Can you work these out from the model? Positions are in its coordinate system, mm. A direction names the side the tool comes from. Round coordinates to 2 decimals unless told otherwise and drop trailing zeros. Order: outer loops, then holes, each group sorted by start corner. A loop starts at its lowest first (then second) coordinate and runs counter-clockwise, first axis right, second up.
from build123d import *

# Parameters (mm, degrees)
SKETCH1_W           = 150
SKETCH1_H           = 20
BOSS_EXTRUDE1_DEPTH = 5
SKETCH3_W           = 150
SKETCH3_H           = 5
BOSS_EXTRUDE2_DEPTH = 15
SKETCH5_R           = 2
CUT_EXTRUDE1_DEPTH  = 152.492574075
SKETCH6_R           = 1.75
CUT_EXTRUDE2_DEPTH  = 153.069063257
SKETCH7_W           = 5
SKETCH7_H           = 20
BOSS_EXTRUDE3_DEPTH = 17
SKETCH8_R           = 1.5
CUT_EXTRUDE3_DEPTH  = 152.492574075
FILLET2_R           = 15


with BuildPart() as part:
    # Sketch1 → Boss-Extrude1 (new body)
    with BuildSketch(Plane(origin=(0, 0, 0), x_dir=(1, 0, 0), z_dir=(0, 1, 0))):
        with Locations((75, 10)):
            Rectangle(SKETCH1_W, SKETCH1_H)
    extrude(amount=-BOSS_EXTRUDE1_DEPTH)

    # Sketch3 → Boss-Extrude2 (add)
    with BuildSketch(Plane(origin=(0, 0, 0), x_dir=(1, 0, 0), z_dir=(0, 1, 0))):
        with Locations((75, 17.5)):
            Rectangle(SKETCH3_W, SKETCH3_H)
    extrude(amount=BOSS_EXTRUDE2_DEPTH)

    # Sketch5 → Cut-Extrude1 (cut, through all)
    with BuildSketch(Plane.XY.offset(-15)):
        with Locations((25, 7.5)):
            Circle(SKETCH5_R)
        with Locations((125, 7.5)):
            Circle(SKETCH5_R)
    extrude(amount=-CUT_EXTRUDE1_DEPTH, mode=Mode.SUBTRACT)

    # Sketch6 → Cut-Extrude2 (cut, through all)
    with BuildSketch(Plane(origin=(0, 0, 0), x_dir=(1, 0, 0), z_dir=(0, 1, 0))):
        with Locations(Location((54.35, 5.75, 0), (0, 0, 270))):
            Circle(SKETCH6_R)
        with Locations(Location((96.7, 8.65, 0), (0, 0, 270))):
            Circle(SKETCH6_R)
    extrude(amount=-CUT_EXTRUDE2_DEPTH, mode=Mode.SUBTRACT)

    # Sketch7 → Boss-Extrude3 (add)
    with BuildSketch(Plane.ZY):
        with Locations((-17.5, 5)):
            Rectangle(SKETCH7_W, SKETCH7_H)
    extrude(amount=BOSS_EXTRUDE3_DEPTH)

    # Sketch8 → Cut-Extrude3 (cut, through all)
    with BuildSketch(Plane.XY.offset(-15)):
        with Locations((-12, 5)):
            Circle(SKETCH8_R)
    extrude(amount=-CUT_EXTRUDE3_DEPTH, mode=Mode.SUBTRACT)

    # Fillet2
    fillet2_edges = [part.edges().sort_by_distance(p)[0] for p in [
        (0, -2.5, -15),
    ]]
    fillet(fillet2_edges, radius=FILLET2_R - 0.0001)  # a hair under: the kernel refuses the full size


solid = part.part
(1) I want a section at C-C, the plane x = 54.35. List the corners of the cut face in (y, z) for me, plus the area to 4 significant figures.
(2) I'm going to push flat-ended pins straight in: pin 1 Ø4.5 at (x, z) = (96.7, -8.65) entering from +Y; pin 2 Ø4 at (x, y) = (125, 7) entering from +Z. Where does each tip first touch, or does it pass through?
(3) I want a section at B-B, the plane y = -2.5. Give the number of separate pieces and of enclosed holes in the cut face, plus the area to 3 significant figures.
(4) Please list where these lines run through material, in increasing order: probe 1 along Y at (x, z) = (-12, -16.6); probe 2 along X at (y, z) = (9, -17.5); probe 3 along Y at (x, z) = (125, -17.95).
(5) I want a section at D-D, the plane z = -13.5. List the corners of the cut face in (x, y) for me.
(6) If we mould it in two halves opening along X, with no side actions, what happens to faces 3 (the face through (-17, 5, -18)), 4 (the face through (23.526, 8.852, -17.465)), 5 (the face through (68, 15, -18))? For each: pulls with the +X half, pulls with the -X half, needs draft (parallel to the pull), parting line crosses it, or undercut.
(7) On a 3-axis mill with a long thin cutter (end or side, diameter ignored), from which of +Z, -Z, +X, -X, +Y, -Y can I reach the whole of each face in a straight line? I mean faces 1 (the face through (66, 0, -8)), 2 (the face through (-4.51, -2.46, -10.72)). Say none if no direction works.
(8) I want a section at A-A, the plane x = 25. List the corners of the cut face in (y, z) for me, plus the area to 3 significant figures.
Ans:
1. outline: (-5, -20) - (15, -20) - (15, -15) - (0, -15) - (0, -7.5) - (-5, -7.5) - close; (-5, -4) - (0, -4) - (0, 0) - (-5, 0) - close
1. area: 157.5 mm2
2. pin 1: stops at y = 0
2. pin 2: stops at z = -15
3. separate pieces: 1
3. enclosed holes: 2
3. area: 3,110 mm2
4. probe 1: y = -5 to 3.5, 6.5 to 15
4. probe 2: x = -17 to 23.68, 26.32 to 123.68, 126.32 to 150
4. probe 3: y = -5 to 5.5, 9.5 to 15
5. outline: (-8.46, -5) - (150, -5) - (150, 0) - (-8.46, 0) - close
6. face 3: pulls with the -X half
6. face 4: undercut
6. face 5: needs draft
7. face 1: +Z, +X, -X, +Y
7. face 2: +Z, -X, +Y, -Y
8. outline: (-5, -20) - (5.5, -20) - (5.5, -15) - (0, -15) - (0, 0) - (-5, 0) - close; (9.5, -20) - (15, -20) - (15, -15) - (9.5, -15) - close
8. area: 155 mm2
